from build123d import *

# Parameters (mm, degrees)
SKETCH_1_W          = 200
SKETCH_1_H          = 146
EXTRUDE_1_DEPTH     = 4
SKETCH_3_R          = 2
CUT_EXTRUDE_1_DEPTH = 202
SKETCH_3_2_R        = 2
SKETCH_3_2_R_2      = 1.5
EXTRUDE_1_2_DEPTH   = 200
SKETCH_4_R          = 2
CUT_EXTRUDE_2_DEPTH = 60
CUT_EXTRUDE_START   = -60
SKETCH_5_R          = 2
CUT_EXTRUDE_3_DEPTH = 60


with BuildPart() as part:
    # 草图1 → Extrude 1 (new body)
    with BuildSketch(Plane(origin=(0, 0, 0), x_dir=(1, 0, 0), z_dir=(0, 1, 0))):
        with Locations((4.739336493, 7.123222749)):
            Rectangle(SKETCH_1_W, SKETCH_1_H)
    extrude(amount=EXTRUDE_1_DEPTH)

    # 草图3 → 切除-拉伸1 (cut)
    with BuildSketch(Plane(origin=(104.739336493, 0, 0), x_dir=(0, 0, -1), z_dir=(1, 0, 0))):
        with Locations((80.123222749, 2)):
            Circle(SKETCH_3_R)
    extrude(amount=-CUT_EXTRUDE_1_DEPTH, mode=Mode.SUBTRACT)

    # 草图3<2> → Extrude 1 2 (add)
    with BuildSketch(Plane(origin=(104.739336493, 0, 0), x_dir=(0, 0, -1), z_dir=(1, 0, 0))):
        with Locations((80.123222749, 2)):
            Circle(SKETCH_3_2_R)
        with Locations((80.123222749, 2)):
            Circle(SKETCH_3_2_R_2, mode=Mode.SUBTRACT)
    extrude(amount=-EXTRUDE_1_2_DEPTH)

    # 草图4 → 切除-拉伸2 (cut)
    with BuildSketch(Plane(origin=(104.739336493, 0, 0), x_dir=(0, 0, -1), z_dir=(1, 0, 0))):
        with Locations((80.123222749, 2)):
            Circle(SKETCH_4_R)
    extrude(amount=-CUT_EXTRUDE_2_DEPTH, mode=Mode.SUBTRACT)

    # 草图5 → 切除-拉伸3 (cut)
    with BuildSketch(Plane.ZY.offset(95.260663507).offset(CUT_EXTRUDE_START)):
        with Locations((-80.123222749, 2)):
            Circle(SKETCH_5_R)
    extrude(amount=CUT_EXTRUDE_3_DEPTH, mode=Mode.SUBTRACT)


solid = part.part
Read the model definition and answer for the solid it produces. Units are mm, in the model's axes. Coordinates: 2 decimals unless noted, no trailing zeros. Loops run counter-clockwise (first coordinate to the right, second up) from the corner with the lowest first, then second, coordinate; pieces in that order, holes last.
Q1. Consider probe 1 along Z at (x, y) = (20.5, 1.7); probe 2 along Z at (x, y) = (88, 1.75); probe 3 along Z at (x, y) = (88, 3). Determine where each line is inside the solid, lowest interval first.
Q2. The part is cut by section A-A on y = 2. Write down the section's boundary in (x, z), and give its area (3 significant figures).
Q3. The part is cut by section B-B on x = -68. Write down the section's boundary in (y, z), and give its area (3 significant figures).
Q4. The mould has two halves that part along Y. Classify faces 1 (the face through (3, 2, 65.877)), 2 (the face through (-64.841, 1.956, -78.124)), 3 (the face through (75.159, 2.044, -78.124)), 4 (the face through (3, 4, -8)): +Y half, -Y half, draft (parallel to the pull), parting line (faces both ways), or undercut.
Q5. Each of these flat-tipped pins is pushed along its axis until it touches: pin 1 Ø2 at (y, z) = (2, -79.5) entering from -X; pin 2 Ø5 at (x, z) = (43, -59) entering from -Y; pin 3 Ø1.2 at (y, z) = (2, -80) entering from +X. Where does it stop, or does it pass through?
Results below:
1. probe 1: z = -82.1 to -81.59, -78.65 to 65.88
1. probe 2: z = -78.14 to 65.88
1. probe 3: z = -78.39 to 65.88
2. outline: (-95.26, -78.12) - (-35.26, -78.12) - (-35.26, -78.62) - (44.74, -78.62) - (44.74, -78.12) - (104.74, -78.12) - (104.74, 65.88) - (-95.26, 65.88) - close; (-35.26, -82.12) - (44.74, -82.12) - (44.74, -81.62) - (-35.26, -81.62) - close
2. area: 28,900 mm2
3. outline: (0, -80.12) arc R2 cw to (4, -80.12) - (4, 65.88) - (0, 65.88) - close
3. area: 578 mm2
4. face 1: draft
4. face 2: undercut
4. face 3: undercut
4. face 4: +Y half
5. pin 1: stops at x = -35.26
5. pin 2: stops at y = 0
5. pin 3: passes through
